Answer from the drawing. Dimensions are ordinates in mm from the lowest x, y and z of the part. A direction names the side the tool comes from. Give positions to 0.01 mm unless a question says otherwise; leave off trailing zeros. Write each loop counter-clockwise with the first axis right and the second up, starting at its lowest first coordinate (ties: lowest second). Pieces come first, ordered by that corner, then holes.
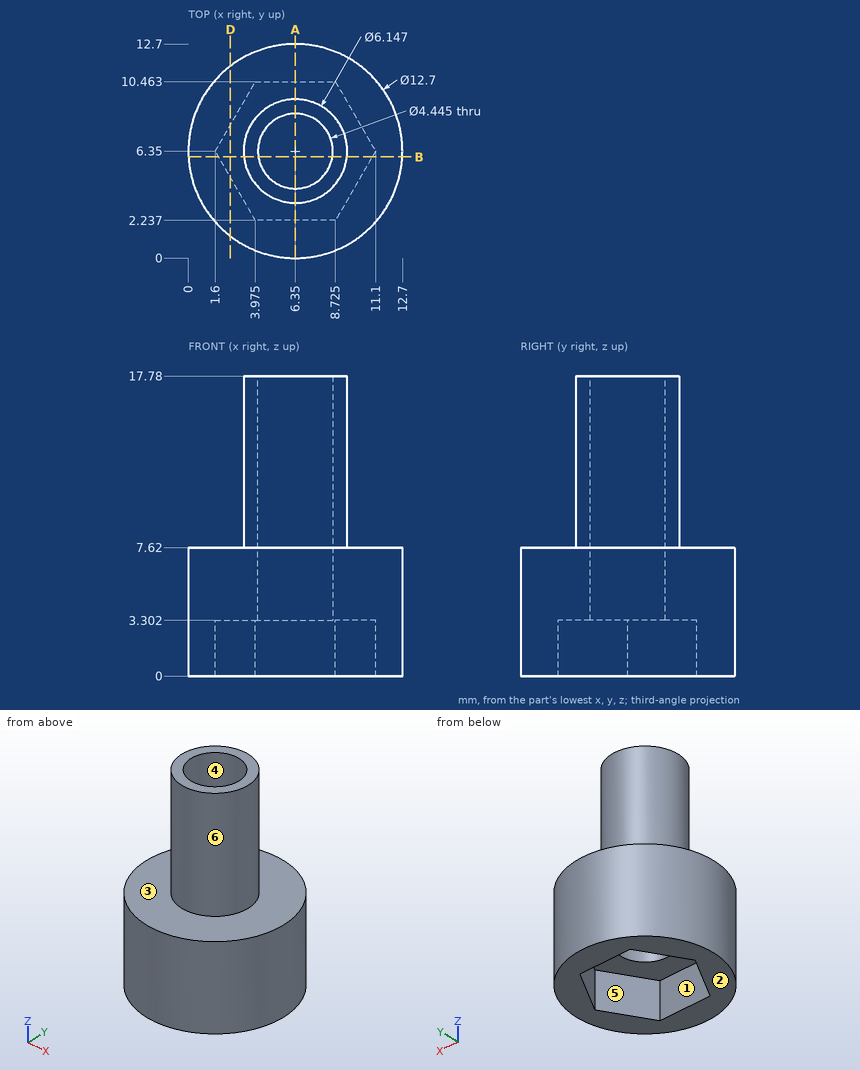
Item 1: Find the intervals of material crossed by line 1 along Y through (x, z) = (6.25, 5.75); line 2 along Y through (x, z) = (6.35, 12), in increasing order.
Result set:
line 1: y = 0 to 4.13, 8.57 to 12.7
line 2: y = 3.28 to 4.13, 8.57 to 9.42
Item 2: Section A-A (x = 6.35) is taken. Write down the section's boundary in (y, z).
Result set:
outline: (0, 0) - (2.24, 0) - (2.24, 3.3) - (4.13, 3.3) - (4.13, 17.78) - (3.28, 17.78) - (3.28, 7.62) - (0, 7.62) - close; (8.57, 3.3) - (10.46, 3.3) - (10.46, 0) - (12.7, 0) - (12.7, 7.62) - (9.42, 7.62) - (9.42, 17.78) - (8.57, 17.78) - close
Item 3: Which of the six approach directions +Z, -Z, +X, -X, +Y, -Y give full straight-line access (tool end or side, diameter ignored) to the marked faces 1 and 2?
Result set:
face 1: -Z
face 2: -Z, +X, -X, +Y, -Y
Item 4: Each of these flat-tipped pins is pushed along its axis until it touches: pin 1 Ø1 at (x, y) = (8.5, 1.5) entering from -Z; pin 2 Ø2 at (y, z) = (3, 6.5) entering from -X; pin 3 Ø1.5 at (y, z) = (3, 9.5) entering from +X; pin 4 Ø4 at (y, z) = (10, 3) entering from -X. Where does it stop, or does it pass through?
Result set:
pin 1: stops at z = 0
pin 2: stops at x = 0.45
pin 3: stops at x = 7.99
pin 4: stops at x = 0.22
Item 5: Section B-B (y = 6) is taken. Write down the section's boundary in (x, z) (1 decimal).
Result set:
outline: (0, 0) - (1.8, 0) - (1.8, 3.3) - (4.2, 3.3) - (4.2, 17.8) - (3.3, 17.8) - (3.3, 7.6) - (0, 7.6) - close; (8.5, 3.3) - (10.9, 3.3) - (10.9, 0) - (12.7, 0) - (12.7, 7.6) - (9.4, 7.6) - (9.4, 17.8) - (8.5, 17.8) - close
Item 6: Section D-D (x = 2.5) is taken. Write down the section's boundary in (y, z).
Result set:
outline: (1.3, 0) - (4.79, 0) - (4.79, 3.3) - (7.91, 3.3) - (7.91, 0) - (11.4, 0) - (11.4, 7.62) - (1.3, 7.62) - close
Item 7: Determine the mould class of the marked faces 3, 4, 5 and 6 for opening direction X: pulls with the +X half, pulls with the -X half, needs draft (parallel to the pull), parting line crosses it, or undercut.
Result set:
face 3: needs draft
face 4: undercut
face 5: undercut
face 6: parting line crosses it
